Could you check a few things on this model? Use its own coordinates, in mm. Face numbers are marked on the shaded views. A direction names the side the tool comes from. Round coordinates to 2 decimals unless told otherwise and drop trailing zeros. Order: outer loops, then holes, each group sorted by start corner. A loop starts at its lowest first (then second) coordinate and runs counter-clockwise, first axis right, second up. Notation, with made-up numbers: (48, 9.5) - (104, 9.5) arc R23 cw to (104, 23.5) - close; hole circle Ø10 at (-14.5, 44.5). An arc over 180 degrees is marked (long way). Use one line per item in the form item = value.
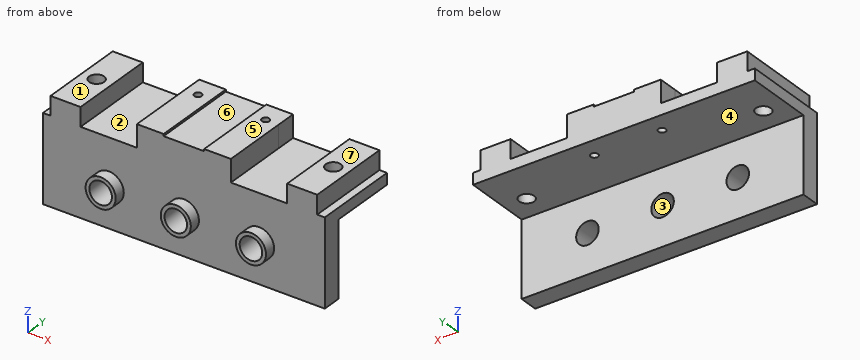
from build123d import *

# Parameters (mm, degrees)
SKETCH1_W            = 50
SKETCH1_H            = 23
BOSS_EXTRUDE12_DEPTH = 3
SKETCH17_W           = 50
SKETCH17_H           = 3
BOSS_EXTRUDE13_DEPTH = 20
BOSS_EXTRUDE15_DEPTH = 25
SKETCH19_R           = 3
CUT_EXTRUDE1_DEPTH   = 10
BOSS_EXTRUDE17_DEPTH = 5.96
CUT_EXTRUDE2_DEPTH   = 58.739515066
SKETCH23_R           = 1
CUT_EXTRUDE3_DEPTH   = 63.190687406
SKETCH24_W           = 8
SKETCH24_H           = 23
BOSS_EXTRUDE20_DEPTH = 5
BOSS_EXTRUDE22_START = 3
SKETCH20_R           = 4
SKETCH20_R_2         = 3
BOSS_EXTRUDE22_DEPTH = 3
SKETCH25_R           = 2
CUT_EXTRUDE4_DEPTH   = 62.749493925
SKETCH26_W           = 75
SKETCH26_H           = 20
BOSS_EXTRUDE23_DEPTH = 2
SKETCH27_R           = 3
CUT_EXTRUDE5_DEPTH   = 57.611408744


with BuildPart() as part:
    # Sketch1 → Boss-Extrude12 (new body)
    with BuildSketch(Plane(origin=(0, 0, 0), x_dir=(1, 0, 0), z_dir=(0, 1, 0))):
        Rectangle(SKETCH1_W, SKETCH1_H)
    extrude(amount=BOSS_EXTRUDE12_DEPTH)

    # Sketch17 → Boss-Extrude13 (add)
    with BuildSketch(Plane(origin=(0, 3, 0), x_dir=(1, 0, 0), z_dir=(0, 1, 0))):
        with Locations((0, -10)):
            Rectangle(SKETCH17_W, SKETCH17_H)
    extrude(amount=BOSS_EXTRUDE13_DEPTH)

    # Sketch18 → Boss-Extrude15 (add)
    with BuildSketch(Plane(origin=(25, 0, 0), x_dir=(0, 0, -1), z_dir=(1, 0, 0))):
        Polygon((-11.5, 23), (-8.5, 23), (-8.5, 3), (11.5, 3), (11.5, 0), (-11.5, 0), align=None)
    extrude(amount=BOSS_EXTRUDE15_DEPTH)

    # Sketch19 → Cut-Extrude1 (cut)
    with BuildSketch(Plane.XZ):
        with Locations(Location((-7.5, -1.069311776, 0), (0, 0, 270))):
            Circle(SKETCH19_R)
        with Locations(Location((12.5, -1.069311776, 0), (0, 0, 270))):
            Circle(SKETCH19_R)
        with Locations(Location((32.5, -1.069311776, 0), (0, 0, 270))):
            Circle(SKETCH19_R)
    extrude(amount=-CUT_EXTRUDE1_DEPTH, mode=Mode.SUBTRACT)

    # Sketch21 → Boss-Extrude17 (add)
    with BuildSketch(Plane.XY.offset(11.5)):
        Polygon((0.022791851, 17.683942334), (0, 0), (25, 0), (24.977208149, 17.683942334), (24.977208149, 23), (0.022791851, 23), align=None)
    extrude(amount=BOSS_EXTRUDE17_DEPTH)

    # Sketch22 → Cut-Extrude2 (cut, through all)
    with BuildSketch(Plane(origin=(0, 23, 0), x_dir=(1, 0, 0), z_dir=(0, 1, 0))):
        Polygon((15.892859801, -16.90901318), (17.890847614, -16.90901318), (17.890847614, -17.46), (7.092859801, -17.46), (7.092859801, -16.90901318), (9.092859801, -16.90901318), align=None)
    extrude(amount=-CUT_EXTRUDE2_DEPTH, mode=Mode.SUBTRACT)

    # Sketch23 → Cut-Extrude3 (cut, through all)
    with BuildSketch(Plane.XY.offset(17.46)):
        with Locations((3.522791851, 17.683942334)):
            Circle(SKETCH23_R)
        with Locations((21.522791851, 17.683942334)):
            Circle(SKETCH23_R)
    extrude(amount=-CUT_EXTRUDE3_DEPTH, mode=Mode.SUBTRACT)

    # Sketch24 → Boss-Extrude20 (add)
    with BuildSketch(Plane.XY.offset(11.5)):
        with Locations((-19, 11.5)):
            Rectangle(SKETCH24_W, SKETCH24_H)
        with Locations((43.983707415, 11.5)):
            Rectangle(SKETCH24_W, SKETCH24_H)
    extrude(amount=BOSS_EXTRUDE20_DEPTH)

    # Sketch20 → Boss-Extrude22 (add)
    # profile 1 of 3: a face of its own
    with BuildSketch(Plane.XZ.offset(BOSS_EXTRUDE22_START)):
        with Locations(Location((-7.5, -1.069311776, 0), (0, 0, 270))):
            Circle(SKETCH20_R)
        with Locations(Location((-7.5, -1.069311776, 0), (0, 0, 270))):
            Circle(SKETCH20_R_2, mode=Mode.SUBTRACT)
    # profile 2 of 3: a face of its own
    with BuildSketch(Plane.XZ.offset(BOSS_EXTRUDE22_START)):
        with Locations(Location((12.5, -1.069311776, 0), (0, 0, 270))):
            Circle(SKETCH20_R)
        with Locations(Location((12.5, -1.069311776, 0), (0, 0, 270))):
            Circle(SKETCH20_R_2, mode=Mode.SUBTRACT)
    # profile 3 of 3: a face of its own
    with BuildSketch(Plane.XZ.offset(BOSS_EXTRUDE22_START)):
        with Locations(Location((32.5, -1.069311776, 0), (0, 0, 270))):
            Circle(SKETCH20_R)
        with Locations(Location((32.5, -1.069311776, 0), (0, 0, 270))):
            Circle(SKETCH20_R_2, mode=Mode.SUBTRACT)
    extrude(amount=-BOSS_EXTRUDE22_DEPTH)

    # Sketch25 → Cut-Extrude4 (cut, through all)
    with BuildSketch(Plane.XY.offset(16.5)):
        with Locations((43.984708093, 11.497259352)):
            Circle(SKETCH25_R)
        with Locations((-19, 11.5)):
            Circle(SKETCH25_R)
    extrude(amount=-CUT_EXTRUDE4_DEPTH, mode=Mode.SUBTRACT)

    # Sketch26 → Boss-Extrude23 (add)
    with BuildSketch(Plane(origin=(0, 3, 0), x_dir=(1, 0, 0), z_dir=(0, 1, 0))):
        with Locations((12.5, 1.5)):
            Rectangle(SKETCH26_W, SKETCH26_H)
    extrude(amount=BOSS_EXTRUDE23_DEPTH)

    # Sketch27 → Cut-Extrude5 (cut, through all)
    with BuildSketch(Plane.XZ.offset(-3)):
        with Locations(Location((-7.5, -1.069311776, 0), (0, 0, 270))):
            Circle(SKETCH27_R)
        with Locations(Location((12.5, -1.069311776, 0), (0, 0, 270))):
            Circle(SKETCH27_R)
        with Locations(Location((32.5, -1.069311776, 0), (0, 0, 270))):
            Circle(SKETCH27_R)
    extrude(amount=-CUT_EXTRUDE5_DEPTH, mode=Mode.SUBTRACT)


solid = part.part
Item 1: Imagine slicing it at A-A on x = -19. Please give me the cut outline in (y, z), plus the area to 3 significant figures.
Found:
outline = (0, -11.5) - (5, -11.5) - (5, 8.5) - (9.5, 8.5) - (9.5, 16.5) - (0, 16.5) - close; (13.5, 8.5) - (23, 8.5) - (23, 16.5) - (13.5, 16.5) - close
area = 252 mm2
Item 2: Imagine slicing it at D-D on y = 0.75. Please give me the cut outline in (x, z).
Found:
outline = (-25, -11.5) - (50, -11.5) - (50, 11.5) - (47.98, 11.5) - (47.98, 16.5) - (39.98, 16.5) - (39.98, 11.5) - (25, 11.5) - (25, 17.46) - (17.89, 17.46) - (17.89, 16.91) - (7.09, 16.91) - (7.09, 17.46) - (0, 17.46) - (0, 11.5) - (-15, 11.5) - (-15, 16.5) - (-23, 16.5) - (-23, 11.5) - (-25, 11.5) - close; hole circle Ø6 at (-7.5, -1.07); hole circle Ø6 at (12.5, -1.07); hole circle Ø6 at (32.5, -1.07)
Item 3: Imagine slicing it at B-B on z = 12.5. Please give me the cut outline in (x, y), plus the area to 3 significant figures.
Found:
outline = (-23, 0) - (-15, 0) - (-15, 23) - (-23, 23) - close; (0, 0) - (25, 0) - (24.98, 17.68) - (24.98, 23) - (0.02, 23) - (0.02, 17.68) - close; (39.98, 0) - (47.98, 0) - (47.98, 23) - (39.98, 23) - close; hole circle Ø4 at (-19, 11.5); hole circle Ø2 at (3.52, 17.68); hole circle Ø2 at (21.52, 17.68); hole circle Ø4 at (43.98, 11.5)
area = 911 mm2
Item 4: For the marked faces 4, 5, 6 and 7, which set-ups out of +Z, -Z, +X, -X, +Y, -Y let a thin tool reach every point of the face, with its end or its side?
Found:
face_4 = -Z, +X, -X, +Y
face_5 = +Z, +X, -X, +Y, -Y
face_6 = +Z, +Y, -Y
face_7 = +Z, +X, +Y, -Y
Item 5: I need wall thicknesses on L1, parallel to X at y = 17.5, z = 9.5; L2, parallel to Z at x = 33.5, y = 8.75; L3, parallel to Y at x = 23.5, z = -3.75. Which ranges of each line are inside material? Lowest first, please.
Found:
L1 = -25 to 2.54, 4.51 to 20.54, 22.51 to 50
L2 = 8.5 to 11.5
L3 = 0 to 5
Item 6: Will these pins go through, and if not, where does the flat tip stop? P1, Ø10, axis at x = 40.5, y = 14.5, coming from the -Z side; P2, Ø8, axis at y = 8, z = 5, coming from the -X side; P3, Ø4, axis at x = 44, y = 11, coming from the +Z side; P4, Ø6, axis at y = 20, z = 15.5, coming from the +X side.
Found:
P1 = 8.5
P2 = -25
P3 = 16.5
P4 = 47.98
Item 7: If we mould it in two halves opening along X, with no side actions, what happens to the marked faces 1, 2 and 3? For each: released by +X, released by -X, zero draft, split by the parting line, or undercut.
Found:
face_1 = zero draft
face_2 = undercut
face_3 = undercut
Item 8: Imagine slicing it at C-C on z = -0.75. Please give me the cut outline in (x, y).
Found:
outline = (-25, 0) - (-11.49, 0) - (-11.49, -3) - (-10.48, -3) - (-10.48, 5) - (-25, 5) - close; (-4.52, -3) - (-3.51, -3) - (-3.51, 0) - (8.51, 0) - (8.51, -3) - (9.52, -3) - (9.52, 5) - (-4.52, 5) - close; (15.48, -3) - (16.49, -3) - (16.49, 0) - (28.51, 0) - (28.51, -3) - (29.52, -3) - (29.52, 5) - (15.48, 5) - close; (35.48, -3) - (36.49, -3) - (36.49, 0) - (50, 0) - (50, 5) - (35.48, 5) - close
